from build123d import *

# Parameters (mm, degrees)
BOSS_EXTRUDE1_DEPTH = 800
FILLET1_R           = 3
FILLET2_R           = 1.5
CHAMFER1_SIZE       = 2


with BuildPart() as part:
    # Sketch1 → Boss-Extrude1 (new body)
    with BuildSketch(Plane(origin=(0, 0, 0), x_dir=(0, 0, -1), z_dir=(1, 0, 0))):
        Polygon((0, 0), (0, 10), (-8, 10), (-8, 8.5), (-1.5, 8.5), (-1.5, 0), align=None)
    extrude(amount=BOSS_EXTRUDE1_DEPTH)

    # Fillet1
    fillet1_edges = [part.edges().sort_by_distance(p)[0] for p in [
        (400, 10, 0),
    ]]
    fillet(fillet1_edges, radius=FILLET1_R)

    # Fillet2
    fillet2_edges = [part.edges().sort_by_distance(p)[0] for p in [
        (400, 8.5, 1.5),
    ]]
    fillet(fillet2_edges, radius=FILLET2_R)

    # Chamfer1
    chamfer1_edges = [part.edges().sort_by_distance(p)[0] for p in [
        (800, 9.25, 8),
        (800, 0, 0.75),
        (0, 9.25, 8),
        (0, 0, 0.75),
    ]]
    chamfer(chamfer1_edges, length=CHAMFER1_SIZE)


solid = part.part
Check sheet for the modelled part. Datum: model origin and axes. Units: mm. Give positions to 0.01 mm unless a question says otherwise; leave off trailing zeros. Write each loop counter-clockwise with the first axis right and the second up, starting at its lowest first coordinate (ties: lowest second). Pieces come first, ordered by that corner, then holes. Notation, with made-up numbers: (28, 46.5) -> (40, 46.5) arc R19 ccw to (40, 63.5) -> close; hole circle Ø11 at (36, -28.5). An arc over 180 degrees is marked (long way). Write item = value, one per line.
Item 1: Sectioned sample at A-A on x = 307. Record the boundary of the cut face in (y, z), and give its area (3 significant figures).
Output:
outline = (0, 0) -> (7, 0) arc R3 ccw to (10, 3) -> (10, 8) -> (8.5, 8) -> (8.5, 3) arc R1.5 cw to (7, 1.5) -> (0, 1.5) -> close
area = 23.3 mm^2
Item 2: Scan lines: probe 1 along Y at (x, z) = (50, 7.5); probe 2 along Z at (x, y) = (624.5, 7); probe 3 along Y at (x, z) = (102, 2.5). Record each from-to range of solid material in increasing order. Write a range as from..to.
Output:
probe_1 = 8.5..10
probe_2 = 0..1.5
probe_3 = 8.41..9.96
Item 3: Gauge pin test, flat ends, axial feed: pin 1 (4 mm diameter, centred on x = 232, z = 6.5, fed in from -Y); pin 2 (2 mm diameter, centred on x = 656, y = 7, fed in from +Z); pin 3 (2 mm diameter, centred on x = 426, y = 5.5, fed in from +Z). Record the tip position at first contact, or that the pin passes through.
Output:
pin_1 = 8.5
pin_2 = 1.88
pin_3 = 1.5
